The model under review builds one solid part; all positions refer to its coordinate system, in mm. A direction names the side the tool comes from. Round coordinates to 2 decimals unless told otherwise and drop trailing zeros. Loops run counter-clockwise (first coordinate to the right, second up) from the corner with the lowest first, then second, coordinate; pieces in that order, holes last. Notation, with made-up numbers: M 50.5,51 L 63.5,51 A30 ccw 63.5,90 Z; hole C -15.75,-6.75 d3. An arc over 180 degrees is marked long. One line per question, with ' | ' between items.
Autodesk Inventor part; units mm, degrees
ref_plane "YZ Plane" through (0, 0, 0) normal (1, 0, 0) x (0, 1, 0)
ref_plane "XZ Plane" through (0, 0, 0) normal (0, 1, 0) x (-1, 0, 0)
ref_plane "XY Plane" through (0, 0, 0) normal (0, 0, 1) x (1, 0, 0)
sketch "Skizze2" plane through (0, 0, 0) normal (0, 1, 0) x (-1, 0, 0)
  line L0 (0, 0) -> (0, -2.5)
  line L1 (0, -2.5) -> (3.2, -2.5)
  arc A0 (15.8, -2.5) -> (3.2, -2.5) centre (9.5, -24.1) ccw
  line L2 (15.8, -2.5) -> (19, -2.5)
  line L3 (19, -2.5) -> (19, 0)
  line L4 (19, 0) -> (0, 0)
  point P0 (9.5, -1.6)
  dimension "d5" = 2.5
  dimension "d6" = 2.5
  dimension "d7" = 3.2
  dimension "d8" = 3.2
  dimension "d9" = 19
  dimension "d10" = 0
  dimension "d11" = 1.6
revolve "Umdrehung2" add sketch "Skizze2" angle 360 about axis through (-19, 0, 0) along (1, 0, 0)
sketch "Skizze3" plane through (-19, 0, 0) normal (-1, 0, 0) x (0, 0, 1)
  line L0 (5, -0.5) -> (-6, -0.5)
  line L1 (-6, -0.5) -> (-6, 0.5)
  line L2 (-6, 0.5) -> (5, 0.5)
  line L3 (5, 0.5) -> (5, -0.5)
  point P0 (0, 0)
  dimension "d13" = 0.5
  dimension "d14" = 0.5
extrude "Extrusion1" cut sketch "Skizze3" against normal blind 1.2
fillet "Rundung1" radius 0.5 4 edges at (-15.8, 0, 2.5) (-19, 2.5, 0) (-19, -2.5, 0) (0, 0, 2.5)
sketch "Skizze4" plane through (0, 0, 0) normal (1, 0, 0) x (0, 0, -1)
  circle A0 centre (0, 0) radius 1.25
  dimension "d18" = 2.5
extrude "Extrusion2" add sketch "Skizze4" along normal blind 25.8
sketch "Skizze5" plane through (25.8, 0, 0) normal (1, 0, 0) x (0, 0, -1)
  circle A0 centre (0, 0) radius 2.4804
  circle A1 centre (0, 0) radius 0.625
  dimension "d21" = 1.25
extrude "Extrusion3" add sketch "Skizze5" along normal blind 176 contours A1
chamfer "Fase1" distance 0.6 distance2 3 1 edges at (201.8, 0, 0.625) measured on face at (201.8, -0.1535, -0.4143)
equation "\"d6\" = d5"
properties part number "Nadel"
1) Insertion check: P1, Ø1.3, axis at x = -18.5, z = -1, coming from the -Y side; P2, Ø1.5, axis at x = 67, y = 1, coming from the +Z side; P3, Ø1.5, axis at x = 6.5, z = 0.5, coming from the +Y side. Each pin has a flat end and moves straight along its axis. Give the tip position at first contact, or say it passes through.
Output values:
P1: stops at y = -2.48 | P2: stops at z = 0.57 | P3: stops at y = 1.25
2) Add section B-B on x = 60. State the section outline as (y, z) points (3 decimals).
Output values:
outline: C 0,0 d1.25
3) Machinability: for faces 1 (the cylindrical face through (-17.204, -0.751, -2.385)), 2 (the flat face through (0, 1, -1)), which of the approach directions +Z, -Z, +X, -X, +Y, -Y give a long, thin tool a straight path to every point of the face, cutting with its end or side? Answer none if there is none.
Output values:
face 1: +X, -X | face 2: +X
4) For line 1 (X direction, y = 1.5, z = 0.25); line 2 (Z direction, x = 144.5, y = -0.4); line 3 (Z direction, x = 101.5, y = -0.05), list the stretches that pass through material, from the lowest coordinate up.
Output values:
line 1: x = -19 to 0 | line 2: z = -0.48 to 0.48 | line 3: z = -0.62 to 0.62
5) Add section A-A on x = 17.5. State the section outline as (y, z) points, then the cut area to 3 significant figures.
Output values:
outline: C 0,0 d2.5 | area: 4.91 mm²
